Source: CAD feature listing. Evaluate the final solid. Frame: model axes, mm. Give positions to 0.01 mm unless a question says otherwise; leave off trailing zeros. Order: outer loops, then holes, each group sorted by start corner. A loop starts at its lowest first (then second) coordinate and runs counter-clockwise, first axis right, second up.
1) Section D-D, the plane x = 109. Return loops of the section in (y, z), plus the area to 3 significant figures.
2) First-contact query: P1, Ø0.6, axis at x = 61, z = 11, coming from the +Y side; P2, Ø0.6, axis at x = 103.5, z = 11.5, coming from the +Y side; P3, Ø0.6, axis at y = 73.5, z = 11, coming from the -X side. Flat tips, straight axial feed; report the tip coordinate or a pass-through.
3) Material intervals for line 1 (X direction, y = 101, z = 11.85); line 2 (X direction, y = 71, z = 11.95); line 3 (X direction, y = 112.5, z = 10.75), sorted ascending.
4) Section A-A, the plane y = 79. Return loops of the section in (x, z).
5) Section C-C, the plane y = 119.5. Return loops of the section in (x, z), plus the area to 3 significant figures.
6) Section B-B, the plane z = 10.6. Give the number of separate pieces and of enclosed holes in the cut face, plus the area to 3 significant figures.
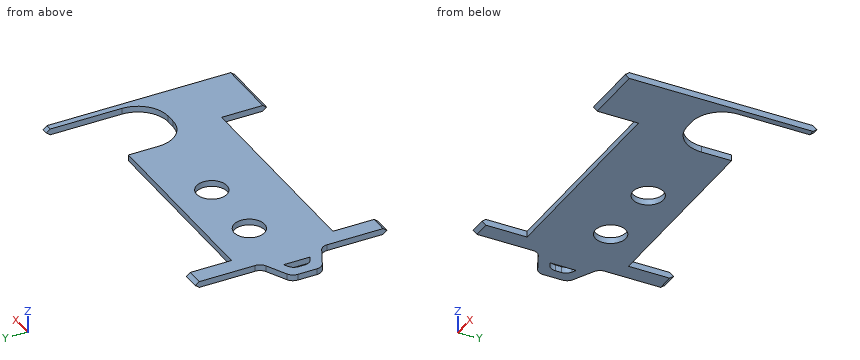
```python
from build123d import *

# Parameters (mm, degrees)
SKETCH1_R           = 5
BOSS_EXTRUDE1_DEPTH = 1
CUT_EXTRUDE1_DEPTH  = 161.089628267
FILLET1_R           = 10
FILLET2_R           = 3


with BuildPart() as part:
    # Sketch1 → Boss-Extrude1 (new, symmetric)
    with BuildSketch(Plane.XY.offset(11.1483132)):
        Polygon((12.416678302, 91.852215255), (22.416678302, 86.852215255), (22.416678302, 65.146170087), (28.004353293, 65.146170087), (28.004353293, 80.146170087), (97.122940581, 80.146170087), (97.122940581, 65.146170087), (117.041628722, 65.146170087), (117.041628722, 128.558260423), (114.975774521, 128.558260423), (114.975774521, 93.558260423), (92.041628722, 93.558260423), (92.041628722, 113.558260423), (28.004353293, 113.558260423), (28.004353293, 128.558260423), (22.416678302, 128.558260423), (22.416678302, 106.852215255), (12.416678302, 101.852215255), align=None)
        Polygon((18.916678302, 92.515334216), (15.916678302, 94.015334216), (15.916678302, 99.689096294), (18.916678302, 101.189096294), align=None, mode=Mode.SUBTRACT)
        with Locations((64.122810805, 100.881519454)):
            Circle(SKETCH1_R, mode=Mode.SUBTRACT)
        with Locations((40.75880907, 100.906977446)):
            Circle(SKETCH1_R, mode=Mode.SUBTRACT)
    extrude(amount=BOSS_EXTRUDE1_DEPTH, both=True)

    # Sketch2 → Cut-Extrude1 (cut, through all)
    with BuildSketch(Plane.ZY.offset(-22.416678302)):
        Polygon((10.106589297, 128.558260423), (10.106589297, 127.082553075), (11.1483132, 128.431101618), (12.190037103, 127.082553075), (12.190037103, 128.558260423), align=None)
        Polygon((12.190037103, 66.621877435), (12.190037103, 65.146170087), (10.106589297, 65.146170087), (10.106589297, 66.621877435), (11.1483132, 65.273328892), align=None)
    extrude(amount=-CUT_EXTRUDE1_DEPTH, mode=Mode.SUBTRACT)

    # Fillet1
    fillet1_edges = [part.edges().sort_by_distance(p)[0] for p in [
        (92.041628722, 93.558260423, 11.1483132),
        (114.975774521, 93.558260423, 11.1483132),
    ]]
    fillet(fillet1_edges, radius=FILLET1_R)

    # Fillet2
    fillet2_edges = [part.edges().sort_by_distance(p)[0] for p in [
        (15.916678302, 94.015334216, 11.1483132),
        (15.916678302, 99.689096294, 11.1483132),
        (22.416678302, 86.852215255, 11.1483132),
        (12.416678302, 91.852215255, 11.1483132),
        (12.416678302, 101.852215255, 11.1483132),
        (22.416678302, 106.852215255, 11.1483132),
    ]]
    fillet(fillet2_edges, radius=FILLET2_R)


solid = part.part
```
From the geometry:
1. outline: (65.27, 11.15) - (66.57, 10.15) - (94.4, 10.15) - (94.4, 12.15) - (66.57, 12.15) - close
1. area: 57.0 mm2
2. P1: stops at y = 113.56
2. P2: stops at y = 93.56
2. P3: stops at x = 22.42
3. line 1: x = 12.59 to 18.54, 18.92 to 35.76, 45.76 to 59.12, 69.12 to 92.37, 114.64 to 117.04
3. line 2: x = 22.42 to 28, 97.12 to 117.04
3. line 3: x = 22.42 to 92.04, 114.98 to 117.04
4. outline: (22.42, 10.15) - (28, 10.15) - (28, 12.15) - (22.42, 12.15) - close; (97.12, 10.15) - (117.04, 10.15) - (117.04, 12.15) - (97.12, 12.15) - close
5. outline: (22.42, 10.15) - (28, 10.15) - (28, 12.15) - (22.42, 12.15) - close; (114.98, 10.15) - (117.04, 10.15) - (117.04, 12.15) - (114.98, 12.15) - close
5. area: 15.3 mm2
6. separate pieces: 1
6. enclosed holes: 3
6. area: 3,190 mm2
